```python
from build123d import *

# Parameters (mm, degrees)
BOSS_EXTRUDE1_DEPTH      = 3
BOSS_EXTRUDE1_DEPTH_BACK = 7
SKETCH1_R                = 10
SKETCH4_R                = 1.6
HOLE_DEPTH               = 19.828402711
HOLECIR_COUNT            = 5
FILLET2_R                = 4


with BuildPart() as part:
    # Sketch1 → Boss-Extrude1 (new, two sides: drawn at the far end of the back side and taken through both)
    with BuildSketch(Plane(origin=(0, 0, 0), x_dir=(1, 0, 0), z_dir=(0, 1, 0)).offset(-BOSS_EXTRUDE1_DEPTH_BACK)):
        with Locations(Location((0, 0, 0), (0, 0, 270))):
            Circle(SKETCH1_R)
    extrude(amount=BOSS_EXTRUDE1_DEPTH + BOSS_EXTRUDE1_DEPTH_BACK)

    # Sketch4 → hole (cut, through all)
    with BuildSketch(Plane(origin=(-3.352872105, -1.093066116, 1.887711608), x_dir=(-0.4486862613641547, -0.14627571033740308, -0.8816371449912632), z_dir=(0.8382180262940947, 0.2732665289126682, -0.47192790187872385))):
        with Locations(Location((0, 0, 0), (0, 0, 8.746528197))):
            Circle(SKETCH4_R)
    hole = extrude(amount=-HOLE_DEPTH, mode=Mode.SUBTRACT)

    # holecir: hole ×5 about axis
    holecir_axis = Axis((0, 0, 0), (0, 1, 0))
    for i in range(1, HOLECIR_COUNT):
        add(hole.rotate(holecir_axis, i * 360 / HOLECIR_COUNT), mode=Mode.SUBTRACT)

    # Fillet2
    # the kernel refuses this fillet: 4 mm, written as the material it takes off along each edge
    with BuildSketch(Plane(origin=(0, -7, 0), x_dir=(0, 0, 1), z_dir=(-1, 0, 0))) as fillet2_piece_1:
        with BuildLine():
            CenterArc((10 - FILLET2_R, FILLET2_R), FILLET2_R, 270, 90)
            Line((10 - FILLET2_R, 0), (10, 0))
            Line((10, 0), (10, FILLET2_R))
        make_face()
    revolve(axis=Axis((0, -7, 0), (0, 1, 0)), mode=Mode.SUBTRACT)
    with BuildSketch(Plane(origin=(0, 3, 0), x_dir=(0, 0, 1), z_dir=(-1, 0, 0))) as fillet2_piece_2:
        with BuildLine():
            CenterArc((10 - FILLET2_R, -FILLET2_R), FILLET2_R, 0, 90)
            Line((10 - FILLET2_R, 0), (10, 0))
            Line((10, 0), (10, -FILLET2_R))
        make_face()
    revolve(axis=Axis((0, 3, 0), (0, 1, 0)), mode=Mode.SUBTRACT)


solid = part.part
```
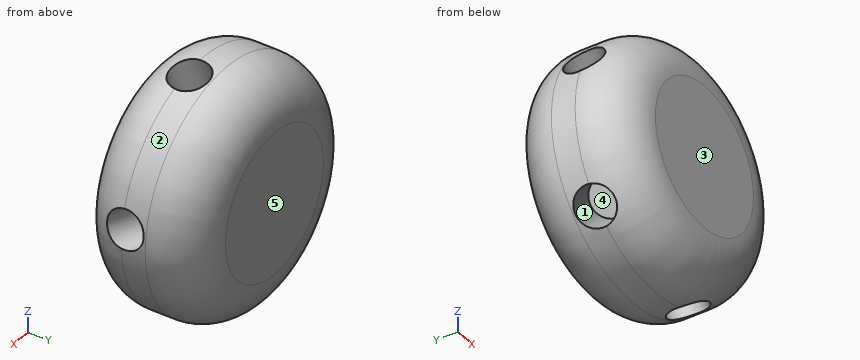
Verification items for the finished model (mm, model axes). Face numbers are marked on the shaded views. A direction names the side the tool comes from. Round coordinates to 2 decimals unless told otherwise and drop trailing zeros. Loops run counter-clockwise (first coordinate to the right, second up) from the corner with the lowest first, then second, coordinate; pieces in that order, holes last. Notation, with made-up numbers: (-5.5, 82) -> (49.5, 82) arc R21 cw to (49.5, 113) -> close; hole circle Ø3 at (59, 45.5). An arc over 180 degrees is marked (long way). Answer as a JSON object with one key per item and string values.
Q1. Draft check along Z on the marked faces 1, 2 and 3. Enter one of: pulls with the +Z half, pulls with the -Z half, needs draft (parallel to the pull), parting line crosses it, or undercut.
Data:
{"face 1": "undercut", "face 2": "parting line crosses it", "face 3": "needs draft"}
Q2. Go/stop test with flat-tipped pins: P1, Ø2, axis at y = -4, z = 7, coming from the -X side; P2, Ø1.5, axis at x = 4, y = -3.5, coming from the +Z side; P3, Ø1, axis at x = -7.5, y = -1, coming from the +Z side. Record where each tip stops, or that it passes through.
Data:
{"P1": "stops at x = -7.89", "P2": "stops at z = 9.39", "P3": "stops at z = 7.14"}
Q3. Section check B-B (x = -3). State how many separate pieces and enclosed holes the cut face has, then the cut area to 3 significant figures.
Data:
{"separate pieces": "1", "enclosed holes": "2", "area": "167 mm2"}
Q4. Access from +Z, -Z, +X, -X, +Y, -Y to the whole of each face (thin tool, end or side, straight path). Record for the marked faces 4 and 5.
Data:
{"face 4": "none", "face 5": "+Z, -Z, +X, -X, +Y"}
Q5. Scan lines: line 1 (Z direction, x = -5.75, y = -1); line 2 (Y direction, x = -5, z = 2); line 3 (X direction, y = -2.5, z = 7.75). Record each from-to range of solid material in increasing order. Write a range as from..to.
Data:
{"line 1": "z = -8.18..-6.4, -3.43..1.54, 4.64..8.18", "line 2": "y = -7..-3.01, -0.03..3", "line 3": "x = -6.32..-0.04, 3.18..6.32"}
Q6. Section check A-A (y = 2). Record the boundary of the cut face in (x, z), then the cut area to 3 significant figures.
Data:
{"outline": "circle Ø17.29 at (0, 0)", "area": "235 mm2"}
